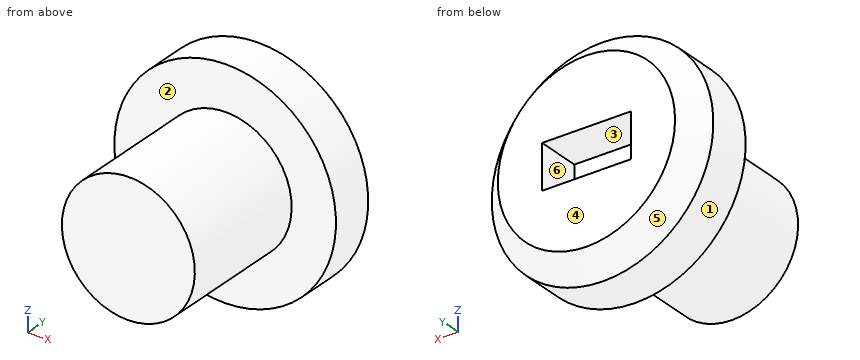
```python
from build123d import *

# Parameters (mm, degrees)
CHAMFER1_SIZE      = 0.5
SKETCH2_W          = 2
SKETCH2_H          = 1
CUT_EXTRUDE1_DEPTH = 1


with BuildPart() as part:
    # Sketch1 → Revolve1 (revolve)
    with BuildSketch(Plane.XY, mode=Mode.PRIVATE) as revolve1_sk:
        Polygon((0, 3.5), (-0.5, 3.5), (-0.5, 4.5), (-2.5, 4.5), (-2.5, 3), (-1.5, 3), (-1.5, 0), (0, 0), align=None)
    revolve(revolve1_sk.sketch.rotate(Axis((0, 0, 0), (0, 1, 0)), 270), axis=Axis((0, 0, 0), (0, 1, 0)))

    # Chamfer1
    chamfer1_edges = [part.edges().sort_by_distance(p)[0] for p in [
        (0, 4.5, 2.5),
    ]]
    chamfer(chamfer1_edges, length=CHAMFER1_SIZE)

    # Sketch2 → Cut-Extrude1 (cut)
    with BuildSketch(Plane(origin=(0, 4.5, 0), x_dir=(1, 0, 0), z_dir=(0, 1, 0))):
        Rectangle(SKETCH2_W, SKETCH2_H)
    extrude(amount=-CUT_EXTRUDE1_DEPTH, mode=Mode.SUBTRACT)


solid = part.part
```
Design review of the part built by this model. Coordinates are the model's own, in mm. Face numbers are marked on the shaded views. A direction names the side the tool comes from. Give positions to 0.01 mm unless a question says otherwise; leave off trailing zeros. Order: outer loops, then holes, each group sorted by start corner. A loop starts at its lowest first (then second) coordinate and runs counter-clockwise, first axis right, second up. Notation, with made-up numbers: (-22, 17) -> (-10, 17) arc R8 ccw to (-10, 32) -> close; hole circle Ø9 at (61, 62.25). An arc over 180 degrees is marked (long way). Write each question's results on one line, items separated by ' | '. Start each with the question number.
Q1. For pin 1 (2 mm diameter, centred on x = -2, z = 1.5, fed in from +Y); pin 2 (0.8 mm diameter, centred on x = 0.5, z = 0, fed in from +Y); pin 3 (1.5 mm diameter, centred on y = 3.5, z = 1, fed in from -X); pin 4 (1 mm diameter, centred on x = 1, y = 1, fed in from -Z), all flat-tipped, find the tip position at first contact; note any pin that passes through.
Q2. Add section A-A on x = 0. Give the boundary of the cut face in (y, z), and give its area (4 significant figures).
Q3. Add section B-B on z = 0. Give the boundary of the cut face in (x, y), and give its area (4 significant figures).
Q4. Machinability: for the marked faces 1 and 2, which of the approach directions +Z, -Z, +X, -X, +Y, -Y give a long, thin tool a straight path to every point of the face, cutting with its end or side? Answer none if there is none.
Q5. Mouldability with a two-part tool opening along X and no side actions: class the marked faces 3, 4, 5 and 6 as +X half, -X half, draft (parallel to the pull), parting line (faces both ways), or undercut.
Q6. Add section C-C on y = 2.6. Give the boundary of the cut face in (x, z).
Q7. Wall thickness on L1, parallel to X at y = 3.9, z = 0.2; L2, parallel to Y at x = -1, z = -1.3; L3, parallel to Z at x = 1.5, y = 3.15: over which ranges is each line inside the solid? List them lowest first. Write a range as from..to.
Found:
1) pin 1: stops at y = 4.5 | pin 2: stops at y = 3.5 | pin 3: stops at x = -2.49 | pin 4: stops at z = -1.41
2) outline: (0, -1.5) -> (3, -1.5) -> (3, -2.5) -> (4, -2.5) -> (4.5, -2) -> (4.5, -0.5) -> (3.5, -0.5) -> (3.5, 0.5) -> (4.5, 0.5) -> (4.5, 2) -> (4, 2.5) -> (3, 2.5) -> (3, 1.5) -> (0, 1.5) -> close | area: 15.25 mm2
3) outline: (-2.5, 3) -> (-1.5, 3) -> (-1.5, 0) -> (1.5, 0) -> (1.5, 3) -> (2.5, 3) -> (2.5, 4) -> (2, 4.5) -> (1, 4.5) -> (1, 3.5) -> (-1, 3.5) -> (-1, 4.5) -> (-2, 4.5) -> (-2.5, 4) -> close | area: 14.25 mm2
4) face 1: +Y, -Y | face 2: -Y
5) face 3: undercut | face 4: draft | face 5: parting line | face 6: undercut
6) outline: circle Ø3 at (0, 0)
7) L1: x = -2.49..-1, 1..2.49 | L2: y = 3..4.5 | L3: z = -2..2
